Here's how the part is built. I have some questions about the finished solid (model axes, mm). Face numbers are marked on the shaded views. Coordinates: 2 decimals unless noted, no trailing zeros. Loops run counter-clockwise (first coordinate to the right, second up) from the corner with the lowest first, then second, coordinate; pieces in that order, holes last. Notation, with made-up numbers: (40.25, -30.75) -> (78.25, -30.75) arc R13 cw to (78.25, -9.75) -> close; hole circle Ø10 at (-26, -25.75). An arc over 180 degrees is marked (long way). Answer as a JSON object with one key per item and string values. Group by question number.
1) I want a section at C-C (x = -16). Write out the boundary of the cut face in (y, z), then the cut area to 3 significant figures.
2) I want a section at B-B (y = 19.5). Write out the boundary of the cut face in (x, z) (3 decimals).
3) I want a section at A-A (z = 10.5). Write out the boundary of the cut face in (x, y).
4) I'm going to push flat-ended pins straight in: pin 1 (10 mm diameter, centred on x = 10.5, z = 4, fed in from +Y); pin 2 (2 mm diameter, centred on x = -46.6, y = 6.13, fed in from -Z); pin 3 (2 mm diameter, centred on y = 33, z = 3.5, fed in from -X); pin 4 (3.5 mm diameter, centred on x = -21.7, y = 41.69, fed in from -Z). Where does each tip first touch, or does it pass through?
5) If we mould it in two halves opening along X, with no side actions, what happens to the marked faces 1, 2 and 3? For each: +X half, -X half, draft (parallel to the pull), parting line (faces both ways), or undercut.
6) I need wall thicknesses on probe 1 along X at (y, z) = (20, 11); probe 2 along X at (y, z) = (22, 12); probe 3 along Y at (x, z) = (4, 9). Which ranges of each line are inside material? Lowest first, please. Write a range as [from, to].
```python
from build123d import *

# Parameters (mm, degrees)
REVOLVE1_ANGLE                  = 180
SKETCH2_W                       = 162.072956604
SKETCH2_H                       = 3.8
CUT_EXTRUDE1_DEPTH              = 19
F_4_40_TAPPED_HOLE1_D           = 2.2606
F_4_40_TAPPED_HOLE1_CSINK_D     = 4.1148
F_4_40_TAPPED_HOLE1_CSINK_ANGLE = 90
CIRPATTERN1_COUNT               = 4
CIRPATTERN1_ANGLE               = 165


with BuildPart() as part:
    # Sketch1 → Revolve1 (revolve, symmetric)
    with BuildSketch(Plane(origin=(0, 0, 0), x_dir=(0, 0, -1), z_dir=(1, 0, 0))) as revolve1_sk:
        Polygon((0, 37), (-18, 37), (-18, 39), (-3, 39), (-3, 42), (-18, 42), (-18, 44), (-3, 44), (-3, 50), (0, 50), align=None)
    revolve(axis=Axis((0, 0, 0), (0, 0, 1)), revolution_arc=REVOLVE1_ANGLE / 2)
    revolve(revolve1_sk.sketch, axis=Axis((0, 0, 0), (0, 0, -1)), revolution_arc=REVOLVE1_ANGLE / 2)

    # Sketch2 → Cut-Extrude1 (cut, through all)
    with BuildSketch(Plane(origin=(0, 0, 0), x_dir=(-1, 0, 0), z_dir=(0, 0, -1))):
        with Locations((0, 1.9)):
            Rectangle(SKETCH2_W, SKETCH2_H)
    extrude(amount=-CUT_EXTRUDE1_DEPTH, mode=Mode.SUBTRACT)

    # #4-40 Tapped Hole1 (through all)
    with Locations(Plane(origin=(0, 0, 0), x_dir=(-1, 0, 0), z_dir=(0, 0, -1))):
        with Locations((-46.597908485, 6.134731034)):
            f_4_40_tapped_hole1 = CounterSinkHole(F_4_40_TAPPED_HOLE1_D / 2, F_4_40_TAPPED_HOLE1_CSINK_D / 2, counter_sink_angle=F_4_40_TAPPED_HOLE1_CSINK_ANGLE)

    # CirPattern1: #4-40 Tapped Hole1 ×4 about axis
    cirpattern1_axis = Axis((0, 0, 0), (0, 0, 1))
    for i in range(1, CIRPATTERN1_COUNT):
        add(f_4_40_tapped_hole1.rotate(cirpattern1_axis, i * CIRPATTERN1_ANGLE / (CIRPATTERN1_COUNT - 1)), mode=Mode.SUBTRACT)


solid = part.part
```
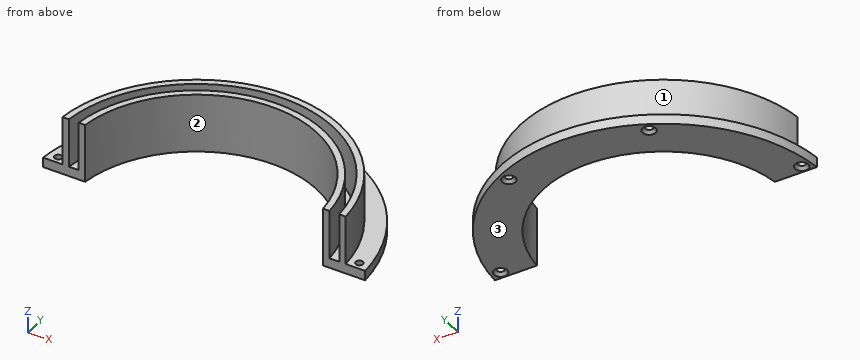
Determined:
{
 "1": {"outline": "(33.36, 0) -> (47.37, 0) -> (47.37, 3) -> (40.99, 3) -> (40.99, 18) -> (38.83, 18) -> (38.83, 3) -> (35.57, 3) -> (35.57, 18) -> (33.36, 18) -> close", "area": "107 mm^2"},
 "2": {"outline": "(-46.041, 0) -> (-31.444, 0) -> (-31.444, 18) -> (-33.775, 18) -> (-33.775, 3) -> (-37.199, 3) -> (-37.199, 18) -> (-39.443, 18) -> (-39.443, 3) -> (-46.041, 3) -> close; (31.444, 0) -> (46.041, 0) -> (46.041, 3) -> (39.443, 3) -> (39.443, 18) -> (37.199, 18) -> (37.199, 3) -> (33.775, 3) -> (33.775, 18) -> (31.444, 18) -> close"},
 "3": {"outline": "(-43.84, 3.8) -> (-41.83, 3.8) arc R42 cw to (41.83, 3.8) -> (43.84, 3.8) arc R44 ccw to start; (-38.81, 3.8) -> (-36.8, 3.8) arc R37 cw to (36.8, 3.8) -> (38.81, 3.8) arc R39 ccw to start"},
 "4": {"pin 1": "y = 49.69", "pin 2": "through", "pin 3": "x = -38.31", "pin 4": "z = 0.31"},
 "5": {"face 1": "parting line", "face 2": "undercut", "face 3": "draft"},
 "6": {"probe 1": "[-39.19, -36.93], [-33.48, -31.13], [31.13, 33.48], [36.93, 39.19]", "probe 2": "[-38.11, -35.78], [-32.2, -29.75], [29.75, 32.2], [35.78, 38.11]", "probe 3": "[36.78, 38.79], [41.81, 43.82]"}
}
